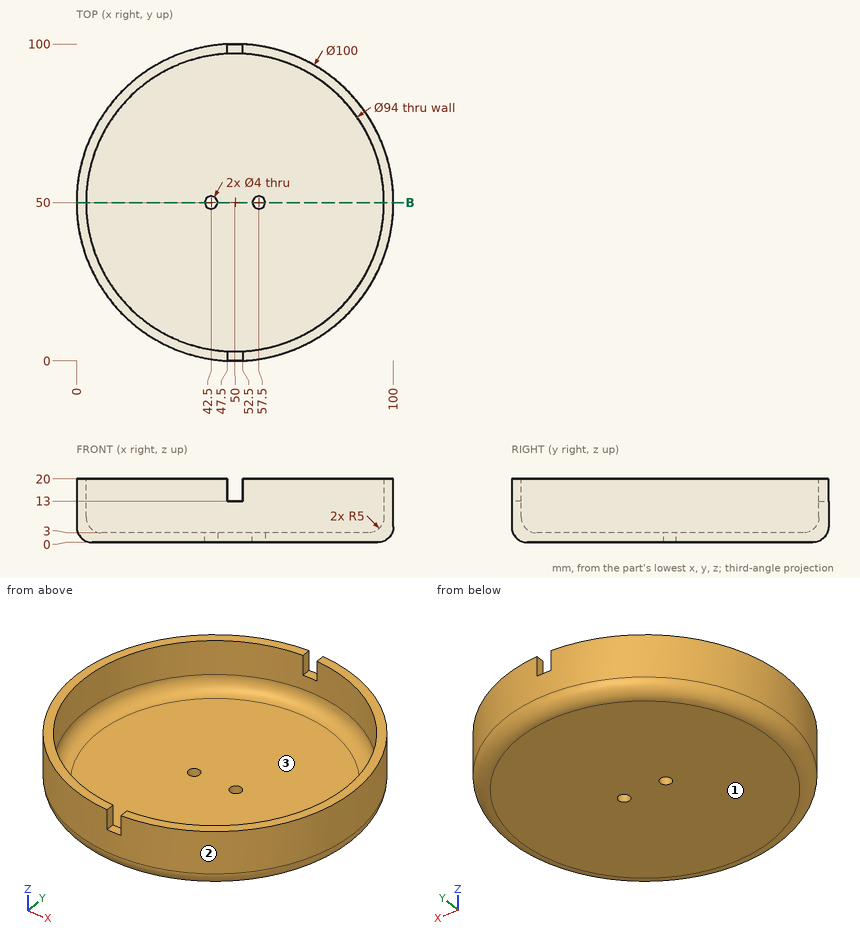
Design review of the part shown in the three views and the two pictorial views. Dimensions are in mm from the part's minimum x, y and z. Coordinates: 2 decimals unless noted, no trailing zeros. One line per question, with ' | ' between items.
Q1. To check wall thickness, follow line 1 along Y through (x, z) = (50, 10.5); line 2 along Y through (x, z) = (57.5, 1.8); line 3 along Z through (x, y) = (19.5, 68). State the ranges of each line that lie inside material, in increasing order.
Answer key:
line 1: y = 0 to 3, 97 to 100 | line 2: y = 1.74 to 48, 52 to 98.26 | line 3: z = 0 to 3
Q2. Clearance check with flat-ended pins moving along their axes: pin 1 Ø12 at (y, z) = (88.5, 12.5) entering from -X; pin 2 Ø4 at (x, z) = (87, 6) entering from -Y; pin 3 Ø1.5 at (y, z) = (45, 6) entering from -X. State where each tip first meets the part, or that it passes through.
Answer key:
pin 1: stops at x = 12 | pin 2: stops at y = 14.29 | pin 3: stops at x = 0.18
Q3. The part is to be moulded in two halves that separate along Y. For the marked faces 1, 2 and 3, say which applies: +Y half, -Y half, draft (parallel to the pull), parting line (faces both ways), or undercut.
Answer key:
face 1: draft | face 2: parting line | face 3: undercut
Q4. Consider section B-B, the plane y = 50. Give the number of separate pieces and of enclosed holes in the cut face, then the cut area to 3 significant figures.
Answer key:
separate pieces: 3 | enclosed holes: 0 | area: 378 mm2
